```python
from build123d import *

# Parameters (mm, degrees)
BOSS_EXTRUDE2_DEPTH  = 4
SKETCH2_R            = 6
BOSS_EXTRUDE3_DEPTH  = 2.5
SKETCH4_R            = 2.5
CUT_EXTRUDE1_DEPTH   = 2.5
LPATTERN1_COUNT      = 3
LPATTERN1_PITCH      = 20
LPATTERN1_COUNT_DIR2 = 6
LPATTERN1_PITCH_DIR2 = 20


with BuildPart() as part:
    # Sketch1 → Boss-Extrude2 (new body)
    with BuildSketch(Plane(origin=(0, 0, 0), x_dir=(1, 0, 0), z_dir=(0, 1, 0))):
        with BuildLine():
            Line((-77.610928287, 24.73480995), (-77.610926739, -10.995486899))
            Line((-77.610926739, -10.995486899), (77.512336703, -10.995486899))
            add(Edge.make_bspline(
                [(77.512336703, -10.995486899), (77.518560385, -10.957874405), (77.524814965, -10.920112686), (77.531107112, -10.882121857)],
                knots=[1.010486637, 1.010486637, 1.010486637, 1.010486637, 1.01412385, 1.01412385, 1.01412385, 1.01412385], degree=3))
            add(Edge.make_bspline(
                [(77.531107112, -10.882121857), (77.574839436, -9.766511083), (77.609892635, -7.507402328), (77.488817492, -4.272864758), (77.205757806, -1.125162749), (76.619514408, 2.937285367), (75.50877626, 7.753752623), (72.989524017, 14.905909338), (68.566776195, 22.780014071), (61.595696469, 30.463398286), (53.335691478, 36.314584962), (44.158321293, 40.264828436), (34.449835996, 42.250559646), (27.85746121, 42.205857253), (24.60638519, 41.843406408)],
                knots=[0.000169226, 0.000169226, 0.000169226, 0.000169226, 0.031413574, 0.062657922, 0.09390227, 0.125146618, 0.187635314, 0.25012401, 0.375101401, 0.500078793, 0.625056185, 0.750033577, 0.875010969, 0.999988361, 0.999988361, 0.999988361, 0.999988361], degree=3))
            add(Edge.make_bspline(
                [(24.60638519, 41.843406408), (19.441654305, 40.599557497), (11.868641969, 38.10186056), (1.706905963, 34.941445063), (-3.490903085, 33.661503777), (-6.113060784, 33.160531214)],
                knots=[0.000658959, 0.000658959, 0.000658959, 0.000658959, 0.498067368, 0.746771573, 0.995475778, 0.995475778, 0.995475778, 0.995475778], degree=3))
            add(Edge.make_bspline(
                [(-6.113060784, 33.160531214), (-7.141691771, 33.016316508), (-9.182526978, 32.742024746), (-13.41706461, 32.236967498), (-18.636406478, 31.76535684), (-24.35525076, 31.602322531), (-29.284430774, 31.960023989), (-33.420361612, 32.921566077), (-36.371506688, 34.261606006), (-38.649706949, 35.648097323), (-40.392953753, 36.835956096), (-41.960752384, 37.950009586), (-43.317594841, 38.899351268), (-44.070083407, 39.410677407), (-44.439121999, 39.658722592)],
                knots=[-0.00019559, -0.00019559, -0.00019559, -0.00019559, 0.062587211, 0.125370012, 0.250935613, 0.376501215, 0.502066816, 0.627632417, 0.753198019, 0.81598082, 0.87876362, 0.941546421, 0.972937821, 1.004329222, 1.004329222, 1.004329222, 1.004329222], degree=3))
            add(Edge.make_bspline(
                [(-44.439121999, 39.658722592), (-44.698278493, 39.837478936), (-45.221943057, 40.202686415), (-46.204449693, 40.903278583), (-47.345032131, 41.729218311), (-48.599765224, 42.619793879), (-50.15090873, 43.651280208), (-51.914572875, 44.618913698), (-53.861511808, 45.22944075), (-55.705524128, 45.327541985), (-57.164765963, 45.050979151), (-58.248551256, 44.683932663), (-59.000335406, 44.361625817), (-59.68368912, 44.01293032), (-60.037538284, 43.806100934), (-60.223947924, 43.693990747)],
                knots=[-0.002497219, -0.002497219, -0.002497219, -0.002497219, 0.029065652, 0.060628523, 0.123754265, 0.186880007, 0.250005749, 0.376257234, 0.502508718, 0.628760202, 0.755011687, 0.818137429, 0.881263171, 0.944388913, 1.007514655, 1.007514655, 1.007514655, 1.007514655], degree=3))
            add(Edge.make_bspline(
                [(-60.223947924, 43.693990747), (-60.647418813, 43.446259773), (-61.492438659, 42.931359573), (-63.090560833, 41.877343183), (-65.712449046, 39.946479206), (-68.970886279, 37.019932698), (-71.698068002, 34.035828956), (-73.643714468, 31.694824796), (-74.523586793, 30.588052824), (-74.969576783, 30.022283972)],
                knots=[0.000174078, 0.000174078, 0.000174078, 0.000174078, 0.062881444, 0.12558881, 0.251003541, 0.501833004, 0.752662466, 0.878077198, 1.003491929, 1.003491929, 1.003491929, 1.003491929], degree=3))
            add(Edge.make_bspline(
                [(-74.969576783, 30.022283972), (-75.519545883, 29.19186114), (-76.530249869, 27.448037515), (-77.287396087, 25.657695857), (-77.610928287, 24.73480995)],
                knots=[0.499549048, 0.499549048, 0.499549048, 0.499549048, 0.499765799, 0.49998255, 0.49998255, 0.49998255, 0.49998255], degree=3))
        make_face()
        with BuildLine():
            Line((77.512336703, -10.995486899), (-77.610926739, -10.995486899))
            Line((-77.610926739, -10.995486899), (-77.610926696, -11.995486899))
            Line((-77.610926696, -11.995486899), (77.352572442, -11.995486899))
            add(Edge.make_bspline(
                [(77.352572442, -11.995486899), (77.358645684, -11.955275612), (77.412259186, -11.602816601), (77.464316371, -11.285695229), (77.512336703, -10.995486899)],
                knots=[0.978851886, 0.978851886, 0.978851886, 0.978851886, 0.982422834, 1.010486637, 1.010486637, 1.010486637, 1.010486637], degree=3))
        make_face()
        with BuildLine():
            Line((77.352572442, -11.995486899), (-77.610926696, -11.995486899))
            Line((-77.610926696, -11.995486899), (-77.610926126, -25.14203309))
            add(Edge.make_bspline(
                [(-77.610926126, -25.14203309), (-77.610329581, -25.399956565), (-77.56299042, -25.903042711), (-77.289715127, -26.985745976), (-76.641681648, -28.530602527), (-75.497775654, -30.448110961), (-73.605831916, -33.039049782), (-70.803315368, -36.111993436), (-67.327412016, -39.127002194), (-64.140223394, -41.243972104), (-61.455644843, -42.436069514), (-59.281170991, -42.877843858), (-58.025592683, -42.909198362), (-57.3728408, -42.946603583)],
                knots=[0.000484301, 0.000484301, 0.000484301, 0.000484301, 0.031521334, 0.062558366, 0.124632431, 0.186706496, 0.248780561, 0.37292869, 0.49707682, 0.62122495, 0.745373079, 0.869521209, 0.993669339, 0.993669339, 0.993669339, 0.993669339], degree=3))
            add(Edge.make_bspline(
                [(-57.3728408, -42.946603583), (-57.13064829, -42.917162583), (-56.655899826, -42.857244252), (-55.632891969, -42.716833971), (-54.283173397, -42.517569574), (-52.529691334, -42.248220025), (-50.028198289, -41.865201142), (-46.600250729, -41.367044153), (-42.036258597, -40.811127611), (-37.051373779, -40.355934431), (-29.881163552, -39.94286355), (-20.010895236, -39.876612938), (-6.937670032, -40.617368244), (4.79101559, -41.816338855), (14.569227449, -42.959318591), (22.067232439, -43.838869966), (29.700051426, -44.671831852), (34.887053568, -45.137323321), (37.472492496, -45.32880882)],
                knots=[0.000538145, 0.000538145, 0.000538145, 0.000538145, 0.016151963, 0.031765781, 0.062993416, 0.094221052, 0.125448688, 0.18790396, 0.250359232, 0.312814503, 0.375269775, 0.500180319, 0.625090862, 0.750001406, 0.812456678, 0.874911949, 0.937367221, 0.999822493, 0.999822493, 0.999822493, 0.999822493], degree=3))
            ThreePointArc((37.472492496, -45.32880882), (38.248733412, -45.324262341), (39.021479233, -45.250543112))
            add(Edge.make_bspline(
                [(39.021479233, -45.250543112), (40.554063275, -45.087269156), (43.636191946, -44.744534775), (49.629747374, -43.872748427), (56.64310661, -42.215757501), (63.76459646, -38.913707507), (69.322535256, -34.215518596), (72.595951354, -29.308690908), (74.463908277, -25.056718438), (75.526739474, -21.803040338), (76.297079472, -18.602211114), (76.745734786, -16.093857572), (77.025988143, -14.25776708), (77.200159766, -13.042150967), (77.304730613, -12.312250405), (77.352572442, -11.995486899)],
                knots=[-0.000308659, -0.000308659, -0.000308659, -0.000308659, 0.063093373, 0.126495404, 0.253299468, 0.380103532, 0.506907596, 0.633711659, 0.697113691, 0.760515723, 0.823917755, 0.887319787, 0.919020803, 0.950721818, 0.978851886, 0.978851886, 0.978851886, 0.978851886], degree=3))
        make_face()
    extrude(amount=BOSS_EXTRUDE2_DEPTH)

    # Sketch2 → Boss-Extrude3 (add)
    with BuildSketch(Plane(origin=(0, 4, 0), x_dir=(1, 0, 0), z_dir=(0, 1, 0))):
        with Locations(Location((-52.601285046, 19.444993701, 0), (0, 0, 270))):
            Circle(SKETCH2_R)
    boss_extrude3 = extrude(amount=BOSS_EXTRUDE3_DEPTH)

    # Sketch4 → Cut-Extrude1 (cut)
    with BuildSketch(Plane(origin=(0, 6.5, 0), x_dir=(1, 0, 0), z_dir=(0, 1, 0))):
        with Locations(Location((-52.601285046, 19.444993701, 0), (0, 0, 270))):
            Circle(SKETCH4_R)
    cut_extrude1 = extrude(amount=-CUT_EXTRUDE1_DEPTH, mode=Mode.SUBTRACT)

    # LPattern1: Boss-Extrude3, Cut-Extrude1 3 × 6
    with Locations(*[(j * LPATTERN1_PITCH_DIR2, 0, i * LPATTERN1_PITCH) for i in range(LPATTERN1_COUNT) for j in range(LPATTERN1_COUNT_DIR2) if (i, j) != (0, 0)]):
        add(boss_extrude3)
        add(cut_extrude1, mode=Mode.SUBTRACT)


solid = part.part
```
Geometry check sheet. Reference: the model listing, model coordinates, mm. A direction names the side the tool comes from. Coordinates: 2 decimals unless noted, no trailing zeros. Use one line per item in the form item = value. Start each with the question number.
1) Go/stop test with flat-tipped pins: pin 1 Ø1.5 at (x, z) = (-53, -0.5) entering from +Y; pin 2 Ø3 at (x, y) = (9, 3) entering from -Z. Record where each tip stops, or that it passes through.
2) Release check for a two-part mould opening along X. For faces 1 (the flat face through (-15, 6.5, 2)), 2 (the cylindrical face through (9.088, 5.268, -1.288)) record: pulls with the +X half, pulls with the -X half, needs draft (parallel to the pull), parting line crosses it, or undercut.
3) Set-up check for faces 3 (the flat face through (-15, 6.5, -18)), 4 (the cylindrical face through (-26.652, 5.232, -0.226)): record each of +Z, -Z, +X, -X, +Y, -Y from which the full face is reachable in a straight line by a thin tool's end or side.
4) Thickness scan on probe 1 along Z at (x, y) = (-53, 5.75); probe 2 along X at (y, z) = (5.75, -4.5); probe 3 along Z at (x, y) = (51, 6). Record the ranges inside material, lowest first. Write a range as from..to.
5) Section check A-A on y = 5.25. State how many separate pieces and enclosed holes the cut face has, and give its area (3 significant figures).
Responses:
q1.pin_1 = 4
q1.pin_2 = -37.7
q2.face_1 = needs draft
q2.face_2 = undercut
q3.face_3 = +Z, -Z, +X, -X, +Y
q3.face_4 = +Y
q4.probe_1 = -25.43..-21.91, -16.98..-13.46, -5.43..-1.91, 3.02..6.54, 14.57..18.09, 23.02..26.54
q4.probe_2 = -55.83..-49.37, -35.83..-29.37, -15.83..-9.37, 4.17..10.63, 24.17..30.63, 44.17..50.63
q4.probe_3 = -24.24..-14.65, -4.24..5.35, 15.76..25.35
q5.separate_pieces = 18
q5.enclosed_holes = 18
q5.area = 1,680 mm2
